```python
from build123d import *

# Parameters (mm, degrees)
HOLE_THREAD_D          = 16.5
HOLE_THREAD_DEPTH      = 7.2
SKETCH5_W              = 14
SKETCH5_H              = 1
EXTRUDE_CUT_DEPTH      = 8
CIRCULAR_PATTERN_COUNT = 6


with BuildPart() as part:
    # Sketch0 → Rotation1 (revolve)
    with BuildSketch(Plane.XY, mode=Mode.PRIVATE) as rotation1_sk:
        Polygon((-12.5, 11.3), (-12.5, 4.3), (-11, 2.8), (-11, 1), (-10, 0), (0, 0), (0, 11.3), align=None)
    revolve(rotation1_sk.sketch.rotate(Axis((0, 0, 0), (0, 1, 0)), 270), axis=Axis((0, 0, 0), (0, 1, 0)))

    # Sketch1 → Revolved Cut1 (revolve, cut)
    with BuildSketch(Plane(origin=(0, 0, 0), x_dir=(0, 0, -1), z_dir=(1, 0, 0)), mode=Mode.PRIVATE) as revolved_cut1_sk:
        Polygon((-5.806624327, 0), (-7.25, 2.5), (-7.25, 4), (-7.192264973, 4.1), (0, 4.1), (0, 0), align=None)
    revolve(revolved_cut1_sk.sketch.rotate(Axis((0, 0, 0), (0, 1, 0)), 180), axis=Axis((0, 0, 0), (0, 1, 0)), mode=Mode.SUBTRACT)

    # Hole/Thread
    with Locations(Plane(origin=(0, 11.3, 0), x_dir=(-1, 0, 0), z_dir=(0, 1, 0))):
        with Locations((0, 0)):
            Hole(HOLE_THREAD_D / 2, depth=HOLE_THREAD_DEPTH)

    # Sketch5 → Extrude Cut (cut)
    with BuildSketch(Plane.XZ):
        with Locations((0, 12)):
            Rectangle(SKETCH5_W, SKETCH5_H)
    extrude_cut = extrude(amount=-EXTRUDE_CUT_DEPTH, mode=Mode.SUBTRACT)

    # Circular Pattern: Extrude Cut ×6 about axis
    circular_pattern_axis = Axis((0, 0, 0), (0, 1, 0))
    for i in range(1, CIRCULAR_PATTERN_COUNT):
        add(extrude_cut.rotate(circular_pattern_axis, i * 360 / CIRCULAR_PATTERN_COUNT), mode=Mode.SUBTRACT)


solid = part.part
```
Check sheet for the modelled part. Datum: model origin and axes. Units: mm. A direction names the side the tool comes from. Give positions to 0.01 mm unless a question says otherwise; leave off trailing zeros. Order: outer loops, then holes, each group sorted by start corner. A loop starts at its lowest first (then second) coordinate and runs counter-clockwise, first axis right, second up. Notation, with made-up numbers: (12, 58) -> (66, 58) arc R32 ccw to (66, 84) -> close; hole circle Ø5 at (74, -3). An arc over 180 degrees is marked (long way). Return JSON: item names as keys, results as strings.
1. Cross-section at A-A, the plane x = 0. Record the cut outline in (y, z).
From the geometry:
{"outline": "(0, -10) -> (1, -11) -> (2.8, -11) -> (3.3, -11.5) -> (8, -11.5) -> (8, -12.5) -> (11.3, -12.5) -> (11.3, -8.25) -> (4.1, -8.25) -> (4.1, -7.19) -> (4, -7.25) -> (2.5, -7.25) -> (0, -5.81) -> close; (0, 5.81) -> (2.5, 7.25) -> (4, 7.25) -> (4.1, 7.19) -> (4.1, 8.25) -> (11.3, 8.25) -> (11.3, 12.5) -> (8, 12.5) -> (8, 11.5) -> (3.3, 11.5) -> (2.8, 11) -> (1, 11) -> (0, 10) -> close"}
2. Go/stop test with flat-tipped pins: P1, Ø4, axis at x = 10, z = 7, coming from the -Y side; P2, Ø0.5, axis at x = 0.5, z = -12, coming from the -Y side; P3, Ø5, axis at x = 5, z = 2, coming from the +Y side. Record where each tip stops, or that it passes through.
From the geometry:
{"P1": "y = 0.21", "P2": "y = 8", "P3": "y = 4.1"}
3. Material ranges on probe 1 along Z at (x, y) = (0, 6.5); probe 2 along Z at (x, y) = (11.5, 10.75); probe 3 along Z at (x, y) = (-4.5, 2.25), recorded low to high. Write a range as [from, to].
From the geometry:
{"probe 1": "[-11.5, -8.25], [8.25, 11.5]", "probe 2": "[-4.9, 4.9]", "probe 3": "[-10.04, -5.5], [5.5, 10.04]"}
4. Set-up check for faces 1 (the flat face through (-10, 8, -6)), 2 (the flat face through (-9.994, 5.617, 5.691)), 3 (the cylindrical face through (7.62, 7.65, -3.16)), 4 (the flat face through (10, 8, -6)), 5 (the flat face through (0, 8, -12)): record each of +Z, -Z, +X, -X, +Y, -Y from which the full face is reachable in a straight line by a thin tool's end or side.
From the geometry:
{"face 1": "-Z, -X, -Y", "face 2": "+Z, -X, -Y", "face 3": "+Y", "face 4": "-Z, +X, -Y", "face 5": "-Z, +X, -X, -Y"}
5. Cross-section at B-B, the plane z = 0. Record the cut outline in (x, y).
From the geometry:
{"outline": "(-12.5, 4.3) -> (-11, 2.8) -> (-11, 1) -> (-10, 0) -> (-5.81, 0) -> (-7.25, 2.5) -> (-7.25, 4) -> (-7.19, 4.1) -> (-8.25, 4.1) -> (-8.25, 11.3) -> (-12.5, 11.3) -> close; (5.81, 0) -> (10, 0) -> (11, 1) -> (11, 2.8) -> (12.5, 4.3) -> (12.5, 11.3) -> (8.25, 11.3) -> (8.25, 4.1) -> (7.19, 4.1) -> (7.25, 4) -> (7.25, 2.5) -> close"}
6. Mould release check, pull along Z, two halves, no side actions. Record for faces 6 (the flat face through (0.6, 4.1, 7.4)), 7 (the cylindrical face through (11.09, 9.31, -5.77)), 8 (the flat face through (9.994, 5.617, -5.691)): +Z half, -Z half, draft (parallel to the pull), parting line (faces both ways), or undercut.
From the geometry:
{"face 6": "undercut", "face 7": "parting line", "face 8": "-Z half"}
